from build123d import *

# Parameters (mm, degrees)
SKETCH1_W           = 152.4
SKETCH1_H           = 152.4
BOSS_EXTRUDE1_DEPTH = 25.4
SKETCH2_W           = 76.2
SKETCH2_H           = 76.2
BOSS_EXTRUDE2_DEPTH = 101.6
CUT_EXTRUDE1_REACH  = 189.083
SKETCH3_R           = 12.7


with BuildPart() as part:
    # Sketch1 → Boss-Extrude1 (new body)
    with BuildSketch(Plane(origin=(0, 0, 0), x_dir=(1, 0, 0), z_dir=(0, 1, 0))):
        Rectangle(SKETCH1_W, SKETCH1_H)
    extrude(amount=BOSS_EXTRUDE1_DEPTH)

    # Sketch2 → Boss-Extrude2 (add)
    with BuildSketch(Plane(origin=(0, 25.4, 0), x_dir=(1, 0, 0), z_dir=(0, 1, 0))):
        Rectangle(SKETCH2_W, SKETCH2_H)
    extrude(amount=BOSS_EXTRUDE2_DEPTH)

    # Sketch3 → Cut-Extrude1 (cut, up to next)
    with BuildSketch(Plane(origin=(38.1, 0, 0), x_dir=(0, 0, -1), z_dir=(1, 0, 0)), mode=Mode.PRIVATE) as cut_extrude1_sk1:
        with Locations((0, 101.6)):
            Circle(SKETCH3_R)
    cut_extrude1_tool1 = extrude(cut_extrude1_sk1.sketch, amount=-CUT_EXTRUDE1_REACH, mode=Mode.PRIVATE) & part.part
    add(cut_extrude1_tool1.solids().sort_by_distance((38.1, 101.6, 0))[0], mode=Mode.SUBTRACT)


solid = part.part
The listing builds one solid part. Answer for the finished solid, in the listing's coordinates (mm). A direction names the side the tool comes from. Coordinates: 2 decimals unless noted, no trailing zeros. Write each loop counter-clockwise with the first axis right and the second up, starting at its lowest first coordinate (ties: lowest second). Pieces come first, ordered by that corner, then holes. Notation, with made-up numbers: M 77.25,56 L 85.25,56 A33 cw 85.25,94 Z; hole C 76.25,58 d11. An arc over 180 degrees is marked long. Put each result on its own line as item: value. Start each with the question number.
1. A cutting plane is placed at D-D on z = -30. Write down the section's boundary in (x, y).
2. For a pull along Z with two mould halves and no side action, classify faces 1 (the flat face through (-1, 13, 76.2)), 2 (the flat face through (-76.2, 13, 1)), 3 (the cylindrical face through (0.533, 114.192, 1.653)) as pulls with the +Z half, pulls with the -Z half, needs draft (parallel to the pull), parting line crosses it, or undercut.
3. A cutting plane is placed at A-A on y = 101.6. Write down the section's boundary in (x, z), then the cut area to 3 significant figures.
4. A cutting plane is placed at B-B on x = 20.5. Write down the section's boundary in (y, z).
5. A cutting plane is placed at C-C on z = 0. Write down the section's boundary in (x, y), then the cut area to 3 significant figures.
6. Consider line 1 (Y direction, x = -5.5, z = 0); line 2 (Z direction, x = -20, y = 101); line 3 (Y direction, x = 52.5, z = 14). Determine where each line is inside the solid, lowest interval first. Write a range as from..to.
7. Flat-ended cylindrical pins translate along their axes: P1, Ø23, axis at x = -18, y = 81, coming from the +Z side; P2, Ø8, axis at y = 100.5, z = 20.5, coming from the +X side; P3, Ø12, axis at y = 56, z = 22, coming from the -X side. Find the tip coordinate at first contact, or state that the pin passes through.
8. Which of the six approach directions +Z, -Z, +X, -X, +Y, -Y give full straight-line access (tool end or side, diameter ignored) to faces 4 (the flat face through (38.1, 75, 1)), 5 (the flat face through (-1, 75, 38.1)), 6 (the flat face through (-38.1, 75, 1))?
Resolved:
1. outline: M -76.2,0 L 76.2,0 L 76.2,25.4 L 38.1,25.4 L 38.1,127 L -38.1,127 L -38.1,25.4 L -76.2,25.4 Z
2. face 1: pulls with the +Z half
2. face 2: needs draft
2. face 3: undercut
3. outline: M -38.1,-38.1 L 38.1,-38.1 L 38.1,-12.7 L -38.1,-12.7 Z; M -38.1,12.7 L 38.1,12.7 L 38.1,38.1 L -38.1,38.1 Z
3. area: 3,870 mm2
4. outline: M 0,-76.2 L 25.4,-76.2 L 25.4,-38.1 L 127,-38.1 L 127,38.1 L 25.4,38.1 L 25.4,76.2 L 0,76.2 Z; hole C 101.6,0 d25.4
5. outline: M -76.2,0 L 76.2,0 L 76.2,25.4 L 38.1,25.4 L 38.1,88.9 L -38.1,88.9 L -38.1,25.4 L -76.2,25.4 Z; M -38.1,114.3 L 38.1,114.3 L 38.1,127 L -38.1,127 Z
5. area: 9,680 mm2
6. line 1: y = 0..88.9, 114.3..127
6. line 2: z = -38.1..-12.69, 12.69..38.1
6. line 3: y = 0..25.4
7. P1: stops at z = 38.1
7. P2: stops at x = 38.1
7. P3: stops at x = -38.1
8. face 4: +Z, -Z, +X, +Y
8. face 5: +Z, +X, -X, +Y
8. face 6: +Z, -Z, -X, +Y
